Read the model definition and answer for the solid it produces. Units are mm, in the model's axes. A direction names the side the tool comes from. Round coordinates to 2 decimals unless told otherwise and drop trailing zeros. Loops run counter-clockwise (first coordinate to the right, second up) from the corner with the lowest first, then second, coordinate; pieces in that order, holes last. Notation, with made-up numbers: (71, 21.5) -> (95, 21.5) arc R28 cw to (95, 47.5) -> close; hole circle Ø6 at (81.25, 2.5). An arc over 180 degrees is marked (long way). Put each result on its own line as item: value.
from build123d import *

# Parameters (mm, degrees)
SKETCH2_W           = 12.6
SKETCH2_H           = 15.2
BOSS_EXTRUDE1_DEPTH = 1
SKETCH3_W           = 11.6
SKETCH3_H           = 14.2
BOSS_EXTRUDE2_DEPTH = 1
SKETCH4_W           = 10.3
SKETCH4_H           = 2.5
CUT_EXTRUDE1_DEPTH  = 4


with BuildPart() as part:
    # Sketch2 → Boss-Extrude1 (new body)
    with BuildSketch(Plane.XY):
        Rectangle(SKETCH2_W, SKETCH2_H)
    extrude(amount=BOSS_EXTRUDE1_DEPTH)

    # Sketch3 → Boss-Extrude2 (add)
    with BuildSketch(Plane(origin=(0, 0, 0), x_dir=(-1, 0, 0), z_dir=(0, 0, -1))):
        Rectangle(SKETCH3_W, SKETCH3_H)
    extrude(amount=BOSS_EXTRUDE2_DEPTH)

    # Sketch4 → Cut-Extrude1 (cut)
    with BuildSketch(Plane(origin=(0, 0, -1), x_dir=(-1, 0, 0), z_dir=(0, 0, -1))):
        with Locations((0, -5.75)):
            Rectangle(SKETCH4_W, SKETCH4_H)
    extrude(amount=-CUT_EXTRUDE1_DEPTH, mode=Mode.SUBTRACT)


solid = part.part
Item 1: The part is cut by section D-D (y = 6.75). Determine the outline of the cut face in (x, z).
Derived:
outline: (-6.3, 0) -> (-5.8, 0) -> (-5.8, -1) -> (5.8, -1) -> (5.8, 0) -> (6.3, 0) -> (6.3, 1) -> (-6.3, 1) -> close
Item 2: Which of the six approach directions +Z, -Z, +X, -X, +Y, -Y give full straight-line access (tool end or side, diameter ignored) to faces 1 (the flat face through (0.1, 7.1, -0.5)), 2 (the flat face through (0.1, -7, 0.2)), 3 (the flat face through (5.8, -0.1, -0.5))?
Derived:
face 1: -Z, +X, -X, +Y
face 2: +Z, -Z
face 3: -Z, +X, +Y, -Y
Item 3: Find the intervals of material crossed by line 1 along Y through (x, z) = (4.75, 0.1); line 2 along X through (y, z) = (3.5, -0.5); line 3 along X through (y, z) = (-5.5, 0.45), in increasing order.
Derived:
line 1: y = -7.6 to -7, -4.5 to 7.6
line 2: x = -5.8 to 5.8
line 3: x = -6.3 to -5.15, 5.15 to 6.3
Item 4: The part is cut by section C-C (x = 0). Determine the outline of the cut face in (y, z).
Derived:
outline: (-7.6, 0) -> (-7.1, 0) -> (-7.1, -1) -> (-7, -1) -> (-7, 1) -> (-7.6, 1) -> close; (-4.5, -1) -> (7.1, -1) -> (7.1, 0) -> (7.6, 0) -> (7.6, 1) -> (-4.5, 1) -> close
Item 5: The part is cut by section A-A (y = -5.5). Determine the outline of the cut face in (x, z), then the cut area to 3 significant figures.
Derived:
outline: (-6.3, 0) -> (-5.8, 0) -> (-5.8, -1) -> (-5.15, -1) -> (-5.15, 1) -> (-6.3, 1) -> close; (5.15, -1) -> (5.8, -1) -> (5.8, 0) -> (6.3, 0) -> (6.3, 1) -> (5.15, 1) -> close
area: 3.60 mm^2
Item 6: For a pull along X with two mould halves and no side action, classify faces 4 (the flat face through (0, 2, -1)), 5 (the flat face through (-5.8, -0.1, -0.5)), 6 (the flat face through (5.15, -6, 0)), 7 (the flat face through (6.3, -0.1, 0.5)) as pulls with the +X half, pulls with the -X half, needs draft (parallel to the pull), parting line crosses it, or undercut.
Derived:
face 4: needs draft
face 5: pulls with the -X half
face 6: undercut
face 7: pulls with the +X half
Item 7: The part is cut by section B-B (z = -0.7). Determine the outline of the cut face in (x, y).
Derived:
outline: (-5.8, -7.1) -> (5.8, -7.1) -> (5.8, 7.1) -> (-5.8, 7.1) -> close; hole (-5.15, -7) -> (5.15, -7) -> (5.15, -4.5) -> (-5.15, -4.5) -> close
